```python
from build123d import *

# Parameters (mm, degrees)
SKETCH1_W           = 44.362146026
SKETCH1_H           = 10
BOSS_EXTRUDE1_DEPTH = 48
SKETCH2_R           = 1.6
CUT_EXTRUDE1_DEPTH  = 27
CUT_EXTRUDE2_START  = -17.925297
SKETCH3_R           = 3.05
CUT_EXTRUDE2_DEPTH  = 12.925297
FILLET1_R           = 3


with BuildPart() as part:
    # Sketch1 → Boss-Extrude1 (new body)
    with BuildSketch(Plane.XY):
        with BuildLine():
            Line((22.181073013, -38), (-22.181073013, -38))
            ThreePointArc((-22.181073013, -38), (0, -44), (22.181073013, -38))
        make_face()
        with BuildLine():
            Line((-37.509998667, -23), (-43.266615306, -23))
            ThreePointArc((-43.266615306, -23), (0, -49), (43.266615306, -23))
            Line((43.266615306, -23), (37.509998667, -23))
            ThreePointArc((37.509998667, -23), (35.812927639, -25.562359318), (33.941125497, -28))
            ThreePointArc((33.941125497, -28), (28.503075122, -33.519765939), (22.181073013, -38))
            ThreePointArc((22.181073013, -38), (0, -44), (-22.181073013, -38))
            ThreePointArc((-22.181073013, -38), (-28.503075122, -33.519765939), (-33.941125497, -28))
            ThreePointArc((-33.941125497, -28), (-35.812927639, -25.562359318), (-37.509998667, -23))
        make_face()
        with BuildLine():
            Line((-29.953929645, -23), (-37.509998667, -23))
            ThreePointArc((-37.509998667, -23), (-35.812927639, -25.562359318), (-33.941125497, -28))
            Line((-33.941125497, -28), (-22.181073013, -28))
            Line((-22.181073013, -28), (-22.181073013, -23))
            Line((-22.181073013, -23), (-29.953929645, -23))
        make_face()
        with BuildLine():
            Line((-22.181073013, -28), (-33.941125497, -28))
            ThreePointArc((-33.941125497, -28), (-28.503075122, -33.519765939), (-22.181073013, -38))
            Line((-22.181073013, -38), (-22.181073013, -28))
        make_face()
        with BuildLine():
            ThreePointArc((33.941125497, -28), (35.812927639, -25.562359318), (37.509998667, -23))
            Line((37.509998667, -23), (22.181073013, -23))
            Line((22.181073013, -23), (22.181073013, -28))
            Line((22.181073013, -28), (33.941125497, -28))
        make_face()
        with BuildLine():
            ThreePointArc((22.181073013, -38), (28.503075122, -33.519765939), (33.941125497, -28))
            Line((33.941125497, -28), (22.181073013, -28))
            Line((22.181073013, -28), (22.181073013, -38))
        make_face()
        with Locations((0, -33)):
            Rectangle(SKETCH1_W, SKETCH1_H)
    extrude(amount=BOSS_EXTRUDE1_DEPTH)

    # Sketch2 → Cut-Extrude1 (cut, through all)
    with BuildSketch(Plane(origin=(0, -23, 0), x_dir=(1, 0, 0), z_dir=(0, 1, 0))):
        with Locations((-29.996615306, -14)):
            Circle(SKETCH2_R)
        with Locations((-29.996615306, -34)):
            Circle(SKETCH2_R)
    cut_extrude1 = extrude(amount=-CUT_EXTRUDE1_DEPTH, mode=Mode.SUBTRACT)

    # Sketch3 → Cut-Extrude2 (cut)
    with BuildSketch(Plane(origin=(0, -23, 0), x_dir=(1, 0, 0), z_dir=(0, 1, 0)).offset(CUT_EXTRUDE2_START)):
        with Locations((-29.996615306, -14)):
            Circle(SKETCH3_R)
        with Locations((-29.996615306, -34)):
            Circle(SKETCH3_R)
    cut_extrude2 = extrude(amount=CUT_EXTRUDE2_DEPTH, mode=Mode.SUBTRACT)

    # Mirror1: Cut-Extrude1, Cut-Extrude2 across plane
    add(cut_extrude1.mirror(Plane(origin=(0, 0, 0), x_dir=(0, 0, 1), z_dir=(1, 0, 0))), mode=Mode.SUBTRACT)
    add(cut_extrude2.mirror(Plane(origin=(0, 0, 0), x_dir=(0, 0, 1), z_dir=(1, 0, 0))), mode=Mode.SUBTRACT)

    # Fillet1
    fillet1_edges = [part.edges().sort_by_distance(p)[0] for p in [
        (-22.181073013, -25.5, 48),
        (-22.181073013, -25.5, 0),
        (0, -28, 0),
        (22.181073013, -23, 24),
        (-22.181073013, -23, 24),
        (-32.723844159, -23, 48),
        (0, -49, 48),
        (32.723844159, -23, 48),
        (22.181073013, -25.5, 48),
        (0, -28, 48),
        (22.181073013, -25.5, 0),
        (32.723844159, -23, 0),
        (0, -49, 0),
        (-32.723844159, -23, 0),
    ]]
    fillet(fillet1_edges, radius=FILLET1_R)


solid = part.part
```
Read the model definition and answer for the solid it produces. Units are mm, in the model's axes. A direction names the side the tool comes from. Coordinates: 2 decimals unless noted, no trailing zeros. Write each loop counter-clockwise with the first axis right and the second up, starting at its lowest first coordinate (ties: lowest second). Pieces come first, ordered by that corner, then holes. Notation, with made-up numbers: (-29, 15) -> (-6, 15) arc R20 ccw to (-6, 21) -> close; hole circle Ø11 at (26.5, 87.25). An arc over 180 degrees is marked (long way). Answer as a JSON object with one key per item and string values.
Q1. A tool of negligible diameter and unlimited length cuts with its end or side. For faces 3 (the flat face through (-28.7, -28, 15.3)), 4 (the cylindrical face through (23.49, -27.98, 47.48)), 5 (the cylindrical face through (-23.04, -23.9, 24.29)), from which of +Z, -Z, +X, -X, +Y, -Y can it reach the whole face along a straight path? Write none if from no direction.
The answers:
{"face 3": "-Y", "face 4": "+Z, +Y", "face 5": "+Z, -Z, +Y"}
Q2. The part is cut by section A-A on z = 6. Give the vertices of the cut face in (x, y), then the cut area to 3 significant figures.
The answers:
{"outline": "(-43.27, -23) arc R49 ccw to (43.27, -23) -> (25.18, -23) arc R3 ccw to (22.18, -26) -> (22.18, -28) -> (-22.18, -28) -> (-22.18, -26) arc R3 ccw to (-25.18, -23) -> close", "area": "1,380 mm2"}
Q3. Determine the mould class of faces 1 (the cylindrical face through (-27.09, -33.12, 13.08)), 2 (the flat face through (-1, -36, 0)) for opening direction X: pulls with the +X half, pulls with the -X half, needs draft (parallel to the pull), parting line crosses it, or undercut.
The answers:
{"face 1": "undercut", "face 2": "needs draft"}
Q4. The part is cut by section C-C on y = -35.5. Give the number of separate pieces and of enclosed holes in the cut face, then the cut area to 3 significant figures.
The answers:
{"separate pieces": "1", "enclosed holes": "4", "area": "3,110 mm2"}
Q5. The part is cut by section B-B on z = 34. Give the vertices of the cut face in (x, y).
The answers:
{"outline": "(-43.27, -23) arc R49 ccw to (-33.05, -36.18) -> (-33.05, -28) -> (-31.6, -28) -> (-31.6, -23) -> close; (-28.4, -28) -> (-26.95, -28) -> (-26.95, -40.93) arc R49 ccw to (26.95, -40.93) -> (26.95, -28) -> (28.4, -28) -> (28.4, -23) -> (25.18, -23) arc R3 ccw to (22.18, -26) -> (22.18, -28) -> (-22.18, -28) -> (-22.18, -26) arc R3 ccw to (-25.18, -23) -> (-28.4, -23) -> close; (31.6, -28) -> (33.05, -28) -> (33.05, -36.18) arc R49 ccw to (43.27, -23) -> (31.6, -23) -> close"}
Q6. Flat-ended cylindrical pins translate along their axes: pin 1 Ø6.5 at (x, z) = (31, 34.5) entering from -Y; pin 2 Ø6 at (x, z) = (-31, 22) entering from -Y; pin 3 Ø1.8 at (x, z) = (30.5, 15) entering from -Y; pin 4 Ø2.5 at (x, z) = (-30, 34) entering from +Y. Find the tip coordinate at first contact, or state that the pin passes through.
The answers:
{"pin 1": "stops at y = -39.76", "pin 2": "stops at y = -40.21", "pin 3": "stops at y = -28", "pin 4": "passes through"}
Q7. Consider line 1 (X direction, y = -27.25, z = 14); line 2 (X direction, y = -25.5, z = 14); line 3 (Y direction, x = -32, z = 15.5). Determine where each line is inside the solid, lowest interval first. Write a range as [from, to].
The answers:
{"line 1": "x = [-40.72, -31.6], [-28.4, -22.18], [22.18, 28.4], [31.6, 40.72]", "line 2": "x = [-41.84, -31.6], [-28.4, -22.22], [22.22, 28.4], [31.6, 41.84]", "line 3": "y = [-28, -23]"}
